Verification items for this drawing (mm, ordinates from the low corner). Coordinates: 2 decimals unless noted, no trailing zeros. Write each loop counter-clockwise with the first axis right and the second up, starting at its lowest first coordinate (ties: lowest second). Pieces come first, ordered by that corner, then holes. Notation, with made-up numbers: (56, 27) -> (75, 27) arc R16 cw to (75, 43) -> close; hole circle Ø5 at (-20, 75.25). An arc over 180 degrees is marked (long way). One line per item, written item: value. Start each with the question number.
1) Sectioned sample at D-D on y = 12.5. Enter the section's corners in (x, z) (1 decimal).
2) Sectioned sample at B-B on x = 20. Enter the section's corners in (y, z).
3) Scan lines: line 1 along Y through (x, z) = (20, 4.5); line 2 along X through (y, z) = (18, 2.7); line 3 along Y through (x, z) = (32.5, 2.55). Record each from-to range of solid material in increasing order. Write a range as [from, to].
4) Draft check along Y on the marked faces 1, 2 and 3. Enter one of: +Y half, -Y half, draft (parallel to the pull), parting line (faces both ways), or undercut.
5) Sectioned sample at A-A on y = 20. Enter the section's corners in (x, z), plus the area to 3 significant figures.
6) Gauge pin test, flat end, axial feed: P1, Ø12, axis at x = 26, y = 25.5, coming from the -Z side. Record the tip position at first contact, or that the pin passes through.
7) Sectioned sample at C-C on z = 1.7. Enter the section's corners in (x, y), plus the area to 3 significant figures.
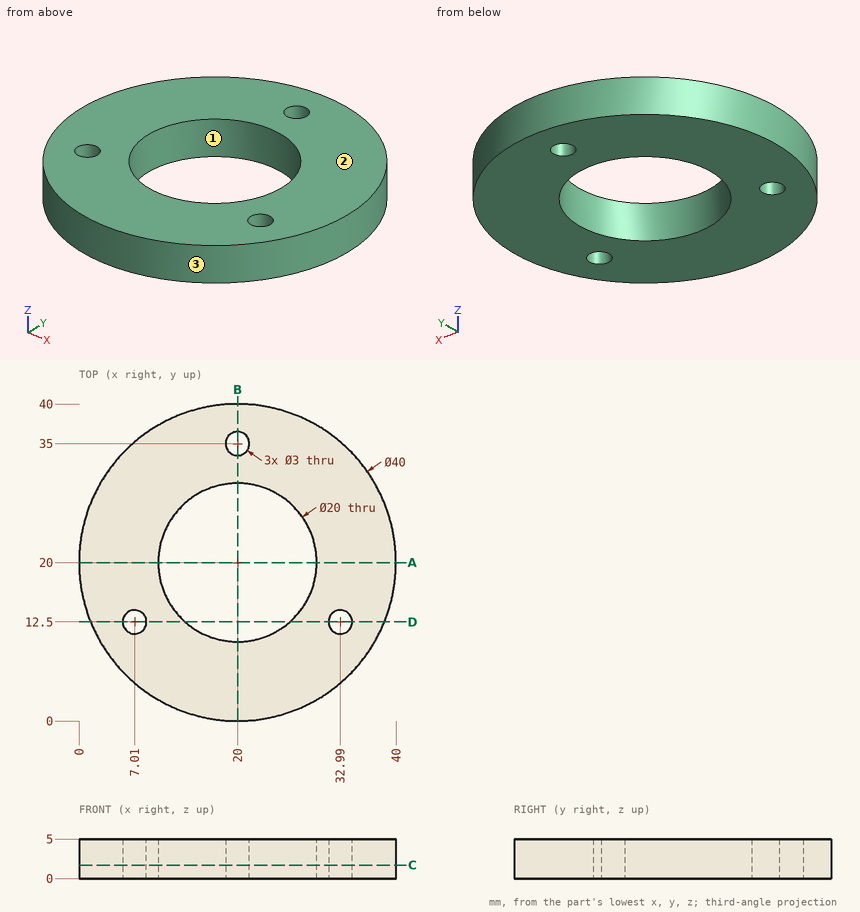
Answers:
1. outline: (1.5, 0) -> (5.5, 0) -> (5.5, 5) -> (1.5, 5) -> close; (8.5, 0) -> (13.4, 0) -> (13.4, 5) -> (8.5, 5) -> close; (26.6, 0) -> (31.5, 0) -> (31.5, 5) -> (26.6, 5) -> close; (34.5, 0) -> (38.5, 0) -> (38.5, 5) -> (34.5, 5) -> close
2. outline: (0, 0) -> (10, 0) -> (10, 5) -> (0, 5) -> close; (30, 0) -> (33.5, 0) -> (33.5, 5) -> (30, 5) -> close; (36.5, 0) -> (40, 0) -> (40, 5) -> (36.5, 5) -> close
3. line 1: y = [0, 10], [30, 33.5], [36.5, 40]
3. line 2: x = [0.1, 10.2], [29.8, 39.9]
3. line 3: y = [4.39, 11.08], [13.92, 35.61]
4. face 1: undercut
4. face 2: draft
4. face 3: parting line
5. outline: (0, 0) -> (10, 0) -> (10, 5) -> (0, 5) -> close; (30, 0) -> (40, 0) -> (40, 5) -> (30, 5) -> close
5. area: 100 mm2
6. P1: stops at z = 0
7. outline: circle Ø40 at (20, 20); hole circle Ø3 at (7.01, 12.5); hole circle Ø20 at (20, 20); hole circle Ø3 at (20, 35); hole circle Ø3 at (32.99, 12.5)
7. area: 921 mm2
